Source: three-view drawing plus pictorial views. Frame: mm from the lowest corner of the part. A direction names the side the tool comes from. Give positions to 0.01 mm unless a question says otherwise; leave off trailing zeros. Order: outer loops, then holes, each group sorted by start corner. A loop starts at its lowest first (then second) coordinate and runs counter-clockwise, first axis right, second up. Notation, with made-up numbers: (75, 34) - (117, 34) arc R29 ccw to (117, 70) - close; hole circle Ø9 at (-35.75, 11.25). An arc over 180 degrees is marked (long way). Answer in a Markdown table with one row per item. Add a question column.
1. Ray query, line 1 (X direction, y = 8.25, z = 6.5); line 2 (Z direction, x = 43, y = 18). Return the intervals inside material, ascending. Write a range as [from, to].
2. Section query B-B on x = 11. Return loops of the section in (y, z).
3. Section query C-C on z = 9. Return loops of the section in (x, y).
4. Contact query for flat-ended pins moving along their axis: pin 1 (7.5 mm diameter, centred on x = 9, y = 14, fed in from +Z); pin 2 (1.5 mm diameter, centred on y = 13.5, z = 10, fed in from -X); pin 3 (6 mm diameter, centred on x = 46, z = 5.5, fed in from -Y); pin 4 (4 mm diameter, centred on y = 8, z = 11.5, fed in from +X). Output: stop coordinate, or through.
5. Section query A-A on y = 5.5. Return loops of the section in (x, z), and give its area (3 significant figures).
6. Access query for the marked faces 1, 2 and 3. Directions: +Z, -Z, +X, -X, +Y, -Y. A direction counts if a zero-diameter tool reaches every point of the face in a straight line with its end or side. Return the directions, or none.
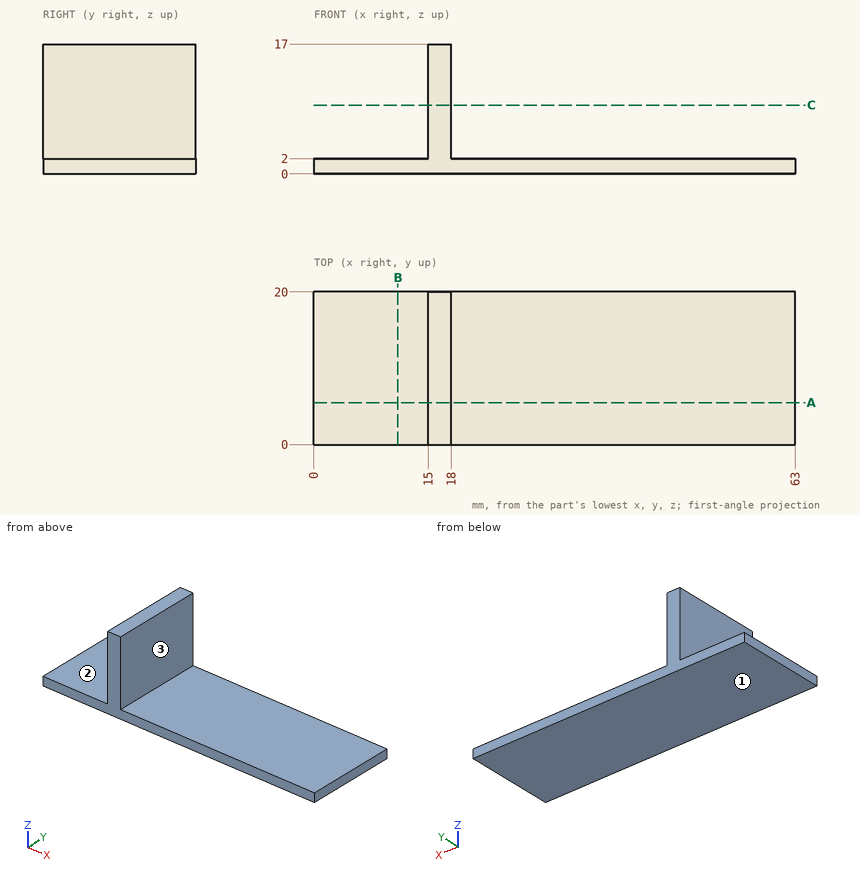
Answer:
| question | item | result |
|---|---|---|
| 1 | line 1 | x = [15, 18] |
| 1 | line 2 | z = [0, 2] |
| 2 | outline | (0, 0) - (20, 0) - (20, 2) - (0, 2) - close |
| 3 | outline | (15, 0) - (18, 0) - (18, 20) - (15, 20) - close |
| 4 | pin 1 | stops at z = 2 |
| 4 | pin 2 | stops at x = 15 |
| 4 | pin 3 | passes through |
| 4 | pin 4 | stops at x = 18 |
| 5 | outline | (0, 0) - (63, 0) - (63, 2) - (18, 2) - (18, 17) - (15, 17) - (15, 2) - (0, 2) - close |
| 5 | area | 171 mm² |
| 6 | face 1 | -Z, +X, -X, +Y, -Y |
| 6 | face 2 | +Z, -X, +Y, -Y |
| 6 | face 3 | +Z, +X, +Y, -Y |
